Model file for the job. Use its own axes, mm. A direction names the side the tool comes from. Coordinates: 2 decimals unless noted, no trailing zeros. Loops run counter-clockwise (first coordinate to the right, second up) from the corner with the lowest first, then second, coordinate; pieces in that order, holes last.
from build123d import *

# Parameters (mm, degrees)
F0_R     = 6.35
F0_W     = 12.7
F0_H     = 25.4
F0_H_2   = 12.7
F1_DEPTH = 12.7
F2_DEPTH = 12.7
F3_DEPTH = 19.05
F4_DEPTH = 12.7
F6_DEPTH = 12.7
F7_R     = 6.34999


# Not quite as in the source:
# - a fillet or chamfer is up to 0.001 mm smaller than in the source, because OpenCascade refuses the exact size


with BuildPart() as f1:
    # F0 (on Top) → F1 (new body)
    with BuildSketch(Plane.XY):
        with BuildLine():
            ThreePointArc((0, -17.2810847643), (19.05, 1.7689152357), (0, 20.8189152357))
            Line((0, 20.8189152357), (-25.4, 20.8189152357))
            Line((-25.4, 20.8189152357), (-25.4, 8.1189152357))
            Line((-25.4, 8.1189152357), (-38.1, 8.1189152357))
            Line((-38.1, 8.1189152357), (-38.1, -17.2810847643))
            Line((-38.1, -17.2810847643), (0, -17.2810847643))
        make_face()
        with Locations((0, 1.7689152357)):
            Circle(F0_R, mode=Mode.SUBTRACT)
        with Locations((-44.45, -4.5810847643)):
            Rectangle(F0_W, F0_H)
        with Locations((-44.45, 14.4689152357)):
            Rectangle(F0_W, F0_H_2)
        with Locations((-31.75, 14.4689152357)):
            Rectangle(F0_W, F0_H_2)
    extrude(amount=F1_DEPTH)

    # F0 (on Top) → F2 (join)
    with BuildSketch(Plane.XY):
        with Locations((-44.45, -4.5810847643)):
            Rectangle(F0_W, F0_H)
        with Locations((-44.45, 14.4689152357)):
            Rectangle(F0_W, F0_H_2)
    extrude(amount=-F2_DEPTH)

    # F0 (on Top) → F3 (join)
    with BuildSketch(Plane.XY):
        with Locations((-31.75, 14.4689152357)):
            Rectangle(F0_W, F0_H_2)
    extrude(amount=F3_DEPTH)

    # F4 (add): a face of the model
    f4_faces = [f1.faces().sort_by_distance(p)[0] for p in [
        (-38.1, 14.4689152357, 15.875),
    ]]
    extrude(f4_faces, amount=F4_DEPTH)

    # F5 (on face) → F6 (join)
    with BuildSketch(Plane.XZ.offset(-8.1189152357)):
        with BuildLine():
            Line((-50.8, 19.05), (-25.4, 19.05))
            ThreePointArc((-25.4, 19.05), (-38.1, 31.75), (-50.8, 19.05))
        make_face()
    extrude(amount=-F6_DEPTH)

    # F7 (radius 6.35 in the source; OpenCascade refuses exactly that, so slightly less here)
    f7_edges = [f1.edges().sort_by_distance(p)[0] for p in [
        (-25.4, 14.468915, 12.7),
    ]]
    fillet(f7_edges, radius=F7_R)


solid = f1.part
Q1. Mould opens along X. For faces 1 (the flat face through (-31, -17.281, 3)), 2 (the cylindrical face through (3.414, 7.123, 6.261)), 3 (the flat face through (-50.8, 2, -1)) say: +X half, -X half, draft (parallel to the pull), parting line (faces both ways), or undercut.
Answers:
face 1: draft
face 2: undercut
face 3: -X half
Q2. Slice it at D-D (z = 10.5). List the corners of the cut face in (x, y), and give its area (3 significant figures).
Answers:
outline: (-50.8, -17.28) - (0, -17.28) arc R19.05 ccw to (0, 20.82) - (-50.8, 20.82) - close; hole circle Ø12.7 at (0, 1.77)
area: 2,380 mm2
Q3. Which spindle directions (+Z, -Z, +X, -X, +Y, -Y) get a long thin tool onto all of the face, cutting with end or side? Do faces 4 (the flat face through (-16, -2, 12.7)), 5 (the flat face through (-10, 2, 0)), 6 (the flat face through (-39, 8.119, 22)). Say none if no direction does.
Answers:
face 4: +Z, +X, -Y
face 5: -Z, +X, +Y, -Y
face 6: +Z, +X, -X, -Y
Q4. Slice it at A-A (x = 2). List the corners of the cut face in (y, z), and give its area (3 significant figures).
Answers:
outline: (-17.18, 0) - (-4.26, 0) - (-4.26, 12.7) - (-17.18, 12.7) - close; (7.8, 0) - (20.71, 0) - (20.71, 12.7) - (7.8, 12.7) - close
area: 328 mm2
Q5. Slice it at C-C (x = -15). List the corners of the cut face in (y, z), and give its area (3 significant figures).
Answers:
outline: (-17.28, 0) - (20.82, 0) - (20.82, 12.7) - (-17.28, 12.7) - close
area: 484 mm2
Q6. Drill centre lines: line 1 (Y direction, x = 0, z = 9.25); line 2 (Y direction, x = -47, z = 17.5); line 3 (X direction, y = 19.5, z = -5). Where is each one in solid material? Low to high.
Answers:
line 1: y = -17.28 to -4.58, 8.12 to 20.82
line 2: y = 8.12 to 20.82
line 3: x = -50.8 to -38.1
Q7. Slice it at B-B (y = -12.5). List the corners of the cut face in (x, z).
Answers:
outline: (-50.8, -12.7) - (-38.1, -12.7) - (-38.1, 0) - (12.62, 0) - (12.62, 12.7) - (-50.8, 12.7) - close
Q8. Flat gauge pins, fed straight in: P1, Ø10, axis at y = 9, z = -9, coming from the +X side; P2, Ø12, axis at y = 5.5, z = 13, coming from the +X side; P3, Ø6, axis at x = 9, y = 6, coming from the +Z side; P4, Ø8, axis at x = -34.5, y = -9.5, coming from the -Z side. Where does each tip first touch, or does it go through?
Answers:
P1: stops at x = -38.1
P2: stops at x = 19.05
P3: stops at z = 12.7
P4: stops at z = -12.7
